```python
from build123d import *

# Parameters (mm, degrees)
F0_R     = 18
F1_DEPTH = 4
F2_R     = 5
F3_D     = 6


with BuildPart() as f1:
    # F0 (on Front) → F1 (new body)
    with BuildSketch(Plane.XZ):
        with BuildLine():
            Line((-12.5, 81.6506350946), (-12.5, 21.6506350946))
            ThreePointArc((-12.5, 21.6506350946), (0, -25), (12.5, 21.6506350946))
            Line((12.5, 21.6506350946), (12.5, 81.6506350946))
            Line((12.5, 81.6506350946), (-12.5, 81.6506350946))
        make_face()
        Circle(F0_R, mode=Mode.SUBTRACT)
    extrude(amount=F1_DEPTH)

    # F2
    f2_edges = [f1.edges().sort_by_distance(p)[0] for p in [
        (12.5, -2, 81.650635),
        (12.5, -2, 21.650635),
        (-12.5, -2, 21.650635),
        (-12.5, -2, 81.650635),
    ]]
    fillet(f2_edges, radius=F2_R)

    # F3 (through all)
    with Locations(Plane(origin=(0, 0, 0), x_dir=(1, 0, 0), z_dir=(0, 1, 0))):
        with Locations((0, -31.6506350946), (0, -71.6506350946)):
            Hole(F3_D / 2)


solid = f1.part
```
Work out the finished part from the listing and answer in its coordinate system (mm). A direction names the side the tool comes from. Coordinates: 2 decimals unless noted, no trailing zeros. Loops run counter-clockwise (first coordinate to the right, second up) from the corner with the lowest first, then second, coordinate; pieces in that order, holes last.
1) Section A-A (z = 0) is taken. Give the vertices of the cut face in (x, y).
Results:
outline: (-25, -4) - (-18, -4) - (-18, 0) - (-25, 0) - close; (18, -4) - (25, -4) - (25, 0) - (18, 0) - close
2) Flat-ended cylindrical pins translate along their axes: pin 1 (2 mm diameter, centred on y = -1.5, z = 41, fed in from +X); pin 2 (8 mm diameter, centred on x = 0, z = 71.65, fed in from -Y); pin 3 (1 mm diameter, centred on y = -3, z = 7.5, fed in from -X); pin 4 (2 mm diameter, centred on y = -1, z = 62, fed in from -X). Find the tip coordinate at first contact, or state that the pin passes through.
Results:
pin 1: stops at x = 12.5
pin 2: stops at y = -4
pin 3: stops at x = -24
pin 4: stops at x = -12.5
3) For faces 4 (the flat face through (12.5, -2, 50)), 5 (the cylindrical face through (0.391, -2.028, 28.676)), 6 (the flat face through (-12.5, -2, 51)), determine the directions among +Z, -Z, +X, -X, +Y, -Y from which every point of the face is accessible in a straight line to the end or side of a thin tool.
Results:
face 4: +Z, +X, +Y, -Y
face 5: +Y, -Y
face 6: +Z, -X, +Y, -Y
4) Section C-C (x = -9.5) is taken. Give the vertices of the cut face in (y, z).
Results:
outline: (-4, -23.12) - (0, -23.12) - (0, -15.29) - (-4, -15.29) - close; (-4, 15.29) - (0, 15.29) - (0, 81.23) - (-4, 81.23) - close
5) Section B-B (x = 0) is taken. Give the vertices of the cut face in (y, z).
Results:
outline: (-4, -25) - (0, -25) - (0, -18) - (-4, -18) - close; (-4, 18) - (0, 18) - (0, 28.65) - (-4, 28.65) - close; (-4, 34.65) - (0, 34.65) - (0, 68.65) - (-4, 68.65) - close; (-4, 74.65) - (0, 74.65) - (0, 81.65) - (-4, 81.65) - close
6) Consider probe 1 along Z at (x, y) = (0, -3.3); probe 2 along X at (y, z) = (-0.4, -11); probe 3 along X at (y, z) = (-2, -15.5). Determine where each line is inside the solid, lowest interval first.
Results:
probe 1: z = -25 to -18, 18 to 28.65, 34.65 to 68.65, 74.65 to 81.65
probe 2: x = -22.45 to -14.25, 14.25 to 22.45
probe 3: x = -19.62 to -9.15, 9.15 to 19.62
7) Section D-D (y = -1.8) is taken. Give the vertices of the cut face in (x, z).
Results:
outline: (-14.58, 20.31) arc R25 ccw (long way) to (14.58, 20.31) arc R5 cw to (12.5, 24.37) - (12.5, 76.65) arc R5 ccw to (7.5, 81.65) - (-7.5, 81.65) arc R5 ccw to (-12.5, 76.65) - (-12.5, 24.37) arc R5 cw to start; hole circle Ø36 at (0, 0); hole circle Ø6 at (0, 31.65); hole circle Ø6 at (0, 71.65)
8) For a pull along X with two mould halves and no side action, classify faces 1 (the cylindrical face through (-2.343, -1.972, 17.847)), 2 (the cylindrical face through (-13.04, -2.03, 22.11)), 3 (the flat face through (0, -2, 81.651)) as +X half, -X half, draft (parallel to the pull), parting line (faces both ways), or undercut.
Results:
face 1: undercut
face 2: -X half
face 3: draft
